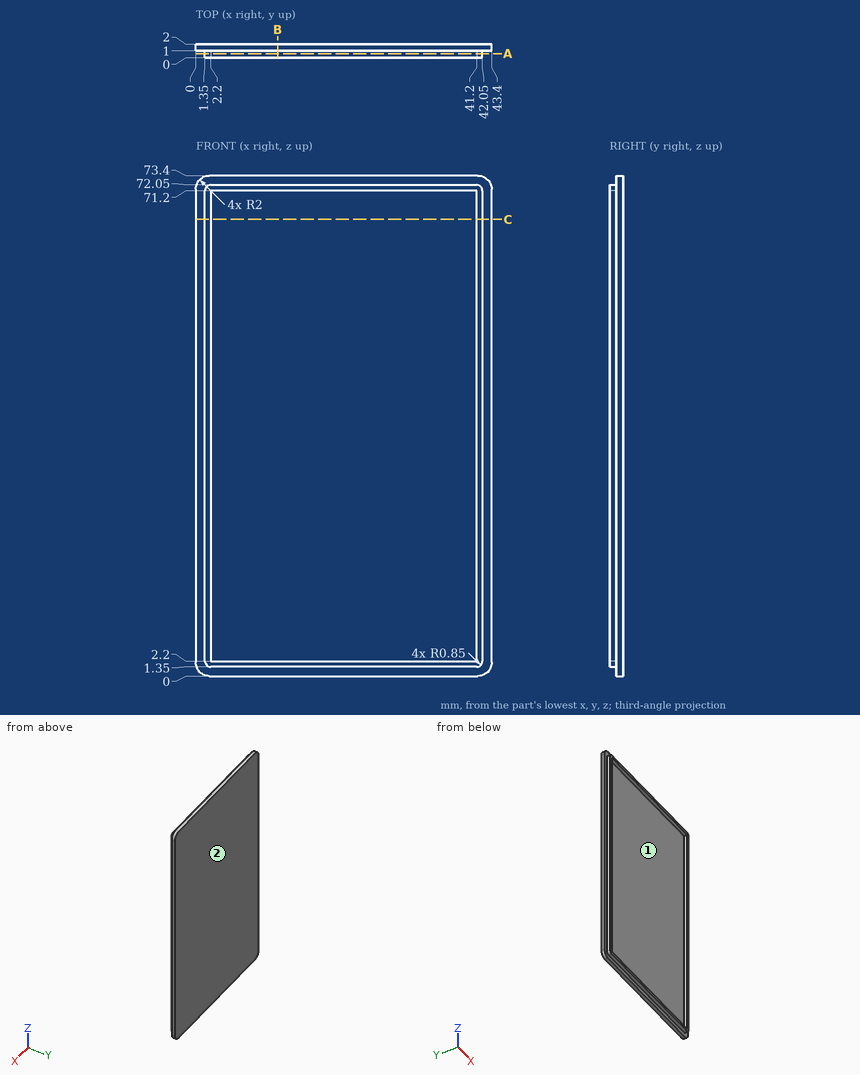
Part print with two shaded views. Sizes in mm from the minimum x, y, z corner. Round coordinates to 2 decimals unless told otherwise and drop trailing zeros. Write each loop counter-clockwise with the first axis right and the second up, starting at its lowest first coordinate (ties: lowest second). Pieces come first, ordered by that corner, then holes. Notation, with made-up numbers: (25.25, -8) -> (41.25, -8) arc R16 cw to (41.25, 20) -> close; hole circle Ø6 at (62.25, -15). An arc over 180 degrees is marked (long way). Put each result on its own line as item: value.
Item 1: Two-plate mould, pull along Z, no slides. Class the marked faces 1 and 2: pulls with the +Z half, pulls with the -Z half, needs draft (parallel to the pull), parting line crosses it, or undercut.
Here are the results:
face 1: undercut
face 2: needs draft
Item 2: Slice it at B-B, the plane x = 12. Give the cut face in (y, z), plus the area to 3 significant figures.
Here are the results:
outline: (0, 1.35) -> (1, 1.35) -> (1, 0) -> (2, 0) -> (2, 73.4) -> (1, 73.4) -> (1, 72.05) -> (0, 72.05) -> (0, 71.2) -> (1, 71.2) -> (1, 2.2) -> (0, 2.2) -> close
area: 75.1 mm^2
Item 3: Slice it at C-C, the plane z = 67. Give the cut face in (x, y), plus the area to 3 significant figures.
Here are the results:
outline: (0, 1) -> (1.35, 1) -> (1.35, 0) -> (2.2, 0) -> (2.2, 1) -> (41.2, 1) -> (41.2, 0) -> (42.05, 0) -> (42.05, 1) -> (43.4, 1) -> (43.4, 2) -> (0, 2) -> close
area: 45.1 mm^2
Item 4: Slice it at A-A, the plane y = 0.6. Give the cut face in (x, z).
Here are the results:
outline: (1.35, 2.2) arc R0.85 ccw to (2.2, 1.35) -> (41.2, 1.35) arc R0.85 ccw to (42.05, 2.2) -> (42.05, 71.2) arc R0.85 ccw to (41.2, 72.05) -> (2.2, 72.05) arc R0.85 ccw to (1.35, 71.2) -> close; hole (2.2, 2.2) -> (41.2, 2.2) -> (41.2, 71.2) -> (2.2, 71.2) -> close
Item 5: Wall check: probe 1 along X at (y, z) = (0.95, 49); probe 2 along Z at (x, y) = (25, 0.75); probe 3 along Y at (x, z) = (5.5, 35). Give the ranges that are in metal, low to high. Write a range as from..to.
Here are the results:
probe 1: x = 1.35..2.2, 41.2..42.05
probe 2: z = 1.35..2.2, 71.2..72.05
probe 3: y = 1..2
Item 6: Flat gauge pins, fed straight in: P1, Ø0.8, axis at x = 19.5, y = 0.5, coming from the -Z side; P2, Ø3, axis at x = 33, z = 27.5, coming from the -Y side; P3, Ø0.5, axis at y = 0.5, z = 44, coming from the +X side. Where does each tip first touch, or does it go through?
Here are the results:
P1: stops at z = 1.35
P2: stops at y = 1
P3: stops at x = 42.05
